from build123d import *

# Parameters (mm, degrees)
F0_R     = 16.860447
F1_DEPTH = 63.5
F2_W     = 20.619992
F2_H     = 58.763284
F3_DEPTH = 25.4
F5_R     = 15.996609
F6_ANGLE = 180


with BuildPart() as f1:
    # F0 (on Front) → F1 (new body)
    with BuildSketch(Plane.XZ):
        with BuildLine():
            Line((-34.240753, -60.200658), (34.240753, -60.200658))
            Line((34.240753, -60.200658), (34.240753, 60.200658))
            ThreePointArc((34.240753, 60.200658), (0, 94.441411), (-34.240753, 60.200658))
            Line((-34.240753, 60.200658), (-34.240753, -60.200658))
        make_face()
        with Locations((0, 60.200658)):
            Circle(F0_R, mode=Mode.SUBTRACT)
    extrude(amount=F1_DEPTH)

    # F2 (on face) → F3 (cut)
    with BuildSketch(Plane.XZ.offset(63.5)):
        Rectangle(F2_W, F2_H)
    extrude(amount=-F3_DEPTH, mode=Mode.SUBTRACT)

    # F5 (on face) → F6 (revolve)
    with BuildSketch(Plane.YZ.offset(34.240753)):
        with Locations((-35.154082, 19.208856)):
            Circle(F5_R)
    revolve(axis=Axis((34.240753, -31.75, -4.22186), (0, 1, 0)), revolution_arc=F6_ANGLE)


solid = f1.part
The model under review builds one solid part; all positions refer to its coordinate system, in mm. A direction names the side the tool comes from. Round coordinates to 2 decimals unless told otherwise and drop trailing zeros. Write each loop counter-clockwise with the first axis right and the second up, starting at its lowest first coordinate (ties: lowest second). Pieces come first, ordered by that corner, then holes. Notation, with made-up numbers: M -11,66 L 6,66 A33 cw 6,98 Z; hole C -16,53.25 d8. An arc over 180 degrees is marked long. Use a Markdown table: item, result. Add a question column.
Q1. We need section C-C, the plane z = 64.5. State the section outline as (x, y) points, plus the area to 3 significant figures.
Q2. The part is to be moulded in two halves that separate along X. For faces 1 (the face through (0, 0, 18)), 2 (the face through (-10.31, -51, 0)), 3 (the face through (-34.241, -31, 1)), say which applies: pulls with the +X half, pulls with the -X half, needs draft (parallel to the pull), parting line crosses it, or undercut.
Q3. We need section B-B, the plane y = -10. State the section outline as (x, z) points.
Q4. To check wall thickness, follow line 1 (Z direction, x = 0, y = -39); line 2 (Z direction, x = 0, y = -24); line 3 (Z direction, x = -6.5, y = -56.5). State the ranges of each line that lie inside material, in increasing order.
Q5. Machinability: for faces 4 (the face through (10.31, -51, 0)), 5 (the face through (-16, -63.5, 18)), which of the approach directions +Z, -Z, +X, -X, +Y, -Y give a long, thin tool a straight path to every point of the face, cutting with its end or side? Answer none if there is none.
Q6. Insertion check: pin 1 (4 mm diameter, centred on x = 40.5, z = 10.5, fed in from -Y); pin 2 (8 mm diameter, centred on x = 45, z = -44.5, fed in from +Y); pin 3 (3 mm diameter, centred on x = 37, y = -36.5, fed in from -Z). Each pin has a flat end and moves straight along its axis. Give the tip position at first contact, or say it passes through.
Q7. We need section A-A, the plane x = 0. State the section outline as (y, z) points.
Findings below:
| question | item | result |
|---|---|---|
| 1 | outline | M -33.97,-63.5 L -16.3,-63.5 L -16.3,0 L -33.97,0 Z; M 16.3,-63.5 L 33.97,-63.5 L 33.97,0 L 16.3,0 Z |
| 1 | area | 2,240 mm² |
| 2 | face 1 | needs draft |
| 2 | face 2 | undercut |
| 2 | face 3 | pulls with the -X half |
| 3 | outline | M -34.24,-60.2 L 34.24,-60.2 L 34.24,60.2 A34.24 ccw -34.24,60.2 Z; hole C 0,60.2 d33.72 |
| 4 | line 1 | z = -60.2 to -29.38, 29.38 to 43.34, 77.06 to 94.44 |
| 4 | line 2 | z = -60.2 to 43.34, 77.06 to 94.44 |
| 4 | line 3 | z = -60.2 to -29.38, 29.38 to 44.64, 75.76 to 93.82 |
| 5 | face 4 | -Y |
| 5 | face 5 | +Z, -Z, +X, -X, -Y |
| 6 | pin 1 | stops at y = -50.2 |
| 6 | pin 2 | stops at y = -27.9 |
| 6 | pin 3 | stops at z = -43.61 |
| 7 | outline | M -63.5,-60.2 L 0,-60.2 L 0,43.34 L -63.5,43.34 L -63.5,29.38 L -38.1,29.38 L -38.1,-29.38 L -63.5,-29.38 Z; M -63.5,77.06 L 0,77.06 L 0,94.44 L -63.5,94.44 Z |
